Could you check a few things on this model? Use its own coordinates, in mm. Face numbers are marked on the shaded views. Coordinates: 2 decimals unless noted, no trailing zeros. Loops run counter-clockwise (first coordinate to the right, second up) from the corner with the lowest first, then second, coordinate; pieces in that order, holes last.
from build123d import *

# Parameters (mm, degrees)
REVOLVE1_ANGLE                  = 180
BOSS_EXTRUDE2_REACH             = 67.818
BOSS_EXTRUDE2_END_RADIUS        = 38
SKETCH2_W                       = 25
SKETCH2_H                       = 35
BOSS_EXTRUDE2_DIRECTION_2_DEPTH = 10
SKETCH5_W                       = 10
SKETCH5_H                       = 120
BOSS_EXTRUDE3_DEPTH             = 7
SKETCH6_W                       = 7
SKETCH6_H                       = 4.5
CUT_EXTRUDE1_DEPTH              = 265


with BuildPart() as part:
    # Sketch1 → Revolve1 (revolve)
    with BuildSketch(Plane.XY):
        with BuildLine():
            Line((0, 38), (0, 33))
            ThreePointArc((0, 33), (33, 0), (0, -33))
            Line((0, -33), (0, -38))
            ThreePointArc((0, -38), (38, 0), (0, 38))
        make_face()
    revolve(axis=Axis((0, -33, 0), (0, -1, 0)), revolution_arc=REVOLVE1_ANGLE)

    # Boss-Extrude2: up to this sphere (the profile starts outside it)
    boss_extrude2_end = Location((0, 0, 0)) * Sphere(BOSS_EXTRUDE2_END_RADIUS, mode=Mode.PRIVATE)
    # Sketch2 → Boss-Extrude2 (add, up to the surface)
    with BuildSketch(Plane(origin=(0, 0, 38), x_dir=(-1, 0, 0), z_dir=(0, 0, -1)), mode=Mode.PRIVATE) as boss_extrude2_sk1:
        Rectangle(SKETCH2_W, SKETCH2_H)
    boss_extrude2_tool1 = extrude(boss_extrude2_sk1.sketch, amount=BOSS_EXTRUDE2_REACH, mode=Mode.PRIVATE) - boss_extrude2_end
    add(boss_extrude2_tool1.solids().sort_by_distance((0, 0, 38))[0])

    # Sketch2 → Boss-Extrude2 direction 2 (add)
    with BuildSketch(Plane(origin=(0, 0, 38), x_dir=(-1, 0, 0), z_dir=(0, 0, -1))):
        Rectangle(SKETCH2_W, SKETCH2_H)
    extrude(amount=-BOSS_EXTRUDE2_DIRECTION_2_DEPTH)

    # Sketch5 → Boss-Extrude3 (add)
    with BuildSketch(Plane.XY.offset(48)):
        with Locations((0, -42.5)):
            Rectangle(SKETCH5_W, SKETCH5_H)
    extrude(amount=-BOSS_EXTRUDE3_DEPTH)

    # Sketch6 → Cut-Extrude1 (cut)
    with BuildSketch(Plane(origin=(0, -102.5, 0), x_dir=(-1, 0, 0), z_dir=(0, -1, 0))):
        with Locations((0, -44.5)):
            Rectangle(SKETCH6_W, SKETCH6_H)
    extrude(amount=-CUT_EXTRUDE1_DEPTH, mode=Mode.SUBTRACT)


solid = part.part
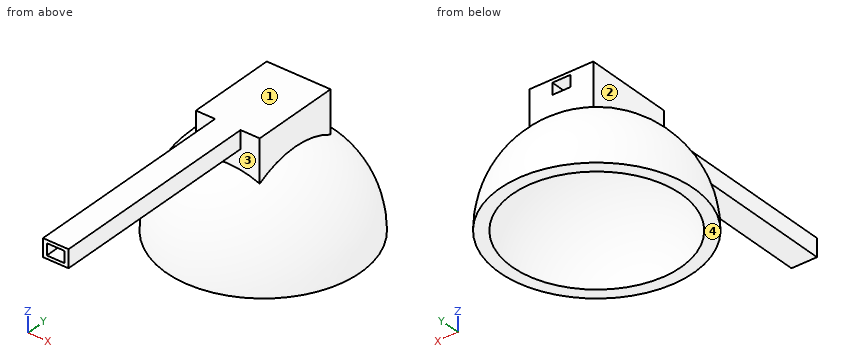
(1) Imagine slicing it at C-C, the plane y = -28. Write out the boundary of the cut face in (x, z).
Answers:
outline: (-25.69, 0) - (-17.46, 0) arc R17.46 cw to (17.46, 0) - (25.69, 0) arc R25.69 ccw to start; (-5, 41) - (5, 41) - (5, 48) - (-5, 48) - close; hole (-3.5, 42.25) - (3.5, 42.25) - (3.5, 46.75) - (-3.5, 46.75) - close
(2) Imagine slicing it at B-B, the plane x = 1.5. Write out the boundary of the cut face in (y, z).
Answers:
outline: (-102.5, 41) - (-17.5, 41) - (-17.5, 33.7) arc R37.97 ccw to (-37.97, 0) - (-32.97, 0) arc R32.97 cw to (32.97, 0) - (37.97, 0) arc R37.97 ccw to (17.5, 33.7) - (17.5, 42.25) - (-102.5, 42.25) - close; (-102.5, 46.75) - (17.5, 46.75) - (17.5, 48) - (-102.5, 48) - close
(3) We'd pull the mould along Z, two halves only. Please class the marked faces 1, 2, 3 and 4: +Z half, -Z half, draft (parallel to the pull), parting line (faces both ways), or undercut.
Answers:
face 1: +Z half
face 2: draft
face 3: undercut
face 4: -Z half
(4) Imagine slicing it at A-A, the plane y = -66. Write out the boundary of the cut face in (x, z), and give its area (3 significant figures).
Answers:
outline: (-5, 41) - (5, 41) - (5, 48) - (-5, 48) - close; hole (-3.5, 42.25) - (3.5, 42.25) - (3.5, 46.75) - (-3.5, 46.75) - close
area: 38.5 mm2
(5) I need wall thicknesses on probe 1 along Y at (x, z) = (-1.5, 8); probe 2 along X at (y, z) = (-57.5, 44); probe 3 along Z at (x, y) = (-0.5, 9.5). Which ranges of each line are inside material? Lowest first, please.
Answers:
probe 1: y = -37.12 to -31.98, 31.98 to 37.12
probe 2: x = -5 to -3.5, 3.5 to 5
probe 3: z = 31.6 to 42.25, 46.75 to 48
(6) For pin 1 (6 mm diameter, centred on y = 13, z = 21.5, fed in from +X); pin 2 (6 mm diameter, centred on x = 25, y = -6, fed in from +Z); pin 3 (1.3 mm diameter, centred on y = -68, z = 45.5, fed in from -X), each with a flat end and sliding along its axis, tell me the tip position at first contact or that it passes through.
Answers:
pin 1: stops at x = 30.89
pin 2: stops at z = 30.47
pin 3: stops at x = -5
(7) Imagine slicing it at D-D, the plane x = 10.5. Write out the boundary of the cut face in (y, z), and give its area (3 significant figures).
Answers:
outline: (-36.52, 0) - (-31.28, 0) arc R31.28 cw to (31.28, 0) - (36.52, 0) arc R36.52 ccw to (17.5, 32.05) - (17.5, 48) - (-17.5, 48) - (-17.5, 32.05) arc R36.52 ccw to start
area: 1,010 mm2
